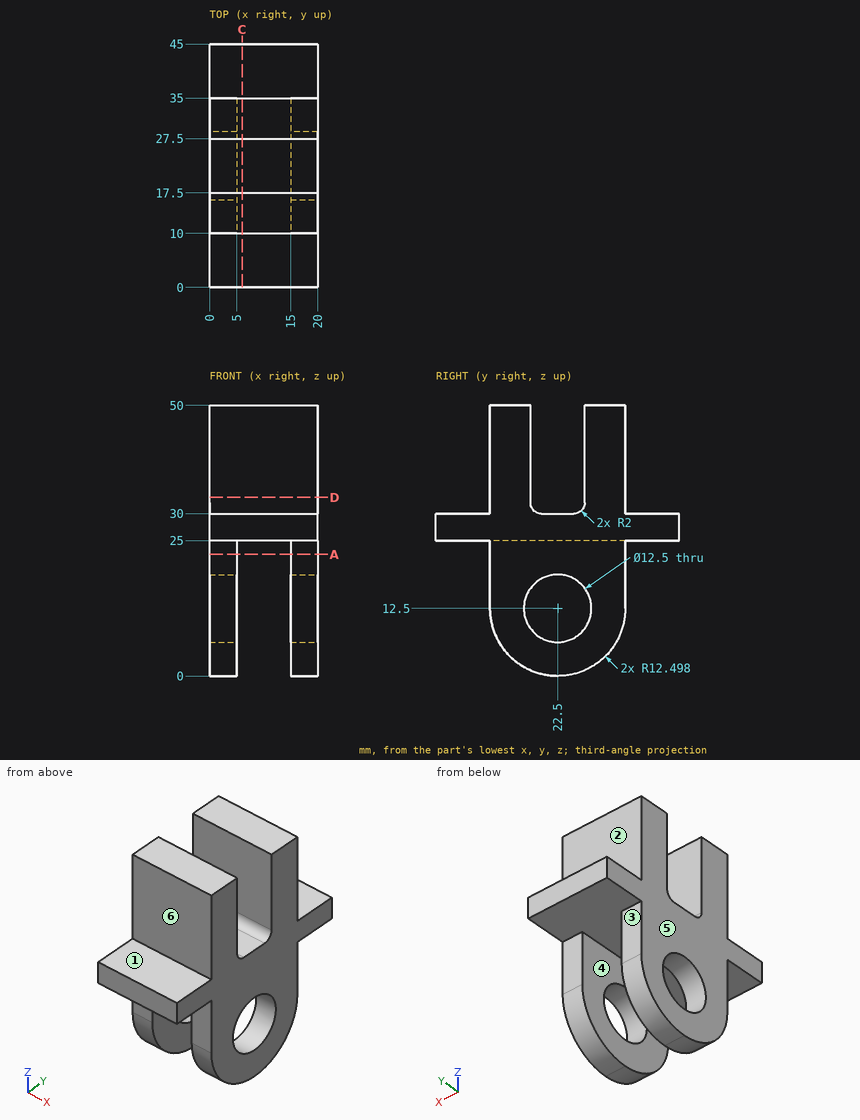
Here's the drawing with two shaded views (mm, measured from the low corner). I have some questions. A direction names the side the tool comes from. Give positions to 0.01 mm unless a question says otherwise; leave off trailing zeros. Order: outer loops, then holes, each group sorted by start corner. A loop starts at its lowest first (then second) coordinate and runs counter-clockwise, first axis right, second up.
Q1. I'm going to push flat-ended pins straight in: P1, Ø11, axis at x = 5.5, y = 41, coming from the +Z side; P2, Ø5.5, axis at x = 17, z = 17.5, coming from the +Y side; P3, Ø6, axis at x = 6.5, z = 36, coming from the -Y side; P4, Ø14.5, axis at y = 22.5, z = 12.5, coming from the -X side. Where does each tip first touch, or does it pass through?
Q2. Suppose I cut it at D-D, the plane z = 33. Write out the boundary of the cut face in (x, y).
Q3. If I drill on line 1 along Z through (x, y) = (18.85, 22.5); line 2 along X through (y, z) = (13.5, 15); line 3 along Y through (x, z) = (5.5, 42), over which ranges is the centre line in solid material (lowest first)?
Q4. For the marked faces 1, 2 and 3, which set-ups out of +Z, -Z, +X, -X, +Y, -Y let a thin tool reach every point of the face, with its end or its side?
Q5. Suppose I cut it at C-C, the plane x = 6. Write out the boundary of the cut face in (y, z).
Q6. Suppose I cut it at A-A, the plane z = 22.5. Write out the boundary of the cut face in (x, y), and give its area (3 significant figures).
Q7. We'd pull the mould along X, two halves only. Please class the marked faces 4, 5 and 6: +X half, -X half, draft (parallel to the pull), parting line (faces both ways), or undercut.
Solution:
1. P1: stops at z = 30
1. P2: stops at y = 35
1. P3: stops at y = 10
1. P4: stops at x = 0
2. outline: (0, 10) - (20, 10) - (20, 17.5) - (0, 17.5) - close; (0, 27.5) - (20, 27.5) - (20, 35) - (0, 35) - close
3. line 1: z = 0 to 6.25, 18.75 to 30
3. line 2: x = 0 to 5, 15 to 20
3. line 3: y = 10 to 17.5, 27.5 to 35
4. face 1: +Z, +X, -X, -Y
4. face 2: +Z, +X, -X, +Y
4. face 3: -Z, +X, -X, +Y
5. outline: (0, 25) - (45, 25) - (45, 30) - (35, 30) - (35, 50) - (27.5, 50) - (27.5, 32) arc R2 cw to (25.5, 30) - (19.5, 30) arc R2 cw to (17.5, 32) - (17.5, 50) - (10, 50) - (10, 30) - (0, 30) - close
6. outline: (0, 10) - (5, 10) - (5, 35) - (0, 35) - close; (15, 10) - (20, 10) - (20, 35) - (15, 35) - close
6. area: 250 mm2
7. face 4: undercut
7. face 5: -X half
7. face 6: draft
